Work out the finished part from the listing and answer in its coordinate system (mm). Face numbers are marked on the shaded views. A direction names the side the tool comes from. Coordinates: 2 decimals unless noted, no trailing zeros. Order: outer loops, then holes, each group sorted by start corner. A loop starts at its lowest first (then second) coordinate and runs counter-clockwise, first axis right, second up. Notation, with made-up numbers: (88.5, -32.5) -> (112.5, -32.5) arc R32 ccw to (112.5, -0.5) -> close; hole circle Ø5 at (88.5, 47.5). An arc over 180 degrees is marked (long way). Answer as CSV lines item,"result". Start each with the question number.
Item 1: Section B-B (z = 1.25) is taken. Write down the section's boundary in (x, y).
Item 2: Section C-C (x = 3.25) is taken. Write down the section's boundary in (y, z).
Item 3: Section A-A (y = 16) is taken. Write down the section's boundary in (x, z), then the cut area to 3 significant figures.
Item 4: Which of the six approach directions +Z, -Z, +X, -X, +Y, -Y give full straight-line access (tool end or side, diameter ignored) to the marked faces 4, 5, 6, 7 and 8?
Item 5: Section D-D (x = -5.25) is taken. Write down the section's boundary in (y, z), then the cut area to 3 significant figures.
Item 6: Each of these flat-tipped pins is pushed along its axis until it touches: pin 1 Ø1.5 at (y, z) = (16, 3) entering from +X; pin 2 Ø3 at (x, y) = (9, 8) entering from -Z; pin 3 Ø4 at (y, z) = (-15, -0.5) entering from -X. Where does it stop, or does it pass through?
Item 7: Straight lines are drawn through the part: L1, parallel to X at y = 13.5, z = 0.25; L2, parallel to X at y = -11.5, z = -1.75; L3, parallel to Y at x = 7.25, z = 0.5. For each, find the intervals that lie inside material, in ascending order.
Item 8: For a pull along X with two mould halves and no side action, classify the marked faces 1, 2 and 3 as pulls with the +X half, pulls with the -X half, needs draft (parallel to the pull), parting line crosses it, or undercut.
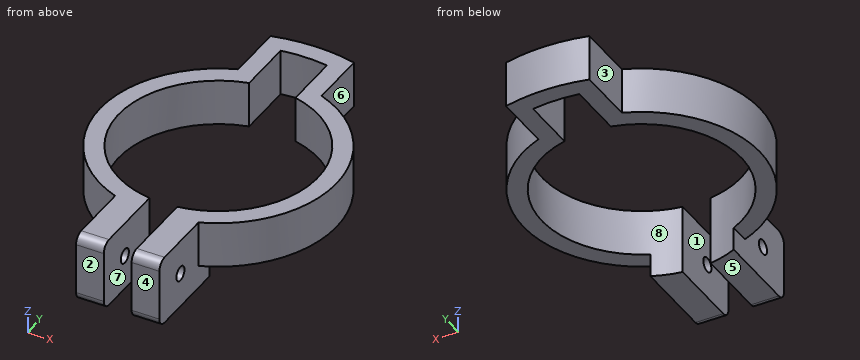
```python
from build123d import *

# Parameters (mm, degrees)
F1_DEPTH = 5
F3_DEPTH = 7.5
F5_DEPTH = 7.5
F6_R     = 1
F7_R     = 0.7847872087
F8_DEPTH = 25


with BuildPart() as f1:
    # F0 (on Top) → F1 (new body)
    with BuildSketch(Plane.XY):
        with BuildLine():
            Line((-4.5, 18.2019916493), (-4.5, 11.9294802904))
            ThreePointArc((-4.5, 11.9294802904), (0, -12.75), (4.5, 11.9294802904))
            Line((4.5, 11.9294802904), (4.5, 18.2019916493))
            ThreePointArc((4.5, 18.2019916493), (0, 18.75), (-4.5, 18.2019916493))
        make_face()
        with BuildLine():
            ThreePointArc((2.5, 10.4552618332), (0, -10.75), (-2.5, 10.4552618332))
            Line((-2.5, 10.4552618332), (-2.5, 16.5623820751))
            ThreePointArc((-2.5, 16.5623820751), (0, 16.75), (2.5, 16.5623820751))
            Line((2.5, 16.5623820751), (2.5, 10.4552618332))
        make_face(mode=Mode.SUBTRACT)
    extrude(amount=F1_DEPTH)

    # F2 (on face) → F3 (join)
    with BuildSketch(Plane.XY.offset(5)):
        with BuildLine():
            ThreePointArc((4.5, -9.7628120949), (0, -10.75), (-4.5, -9.7628120949))
            Line((-4.5, -9.7628120949), (-4.5, -11.9294802904))
            ThreePointArc((-4.5, -11.9294802904), (0, -12.75), (4.5, -11.9294802904))
            Line((4.5, -11.9294802904), (4.5, -9.7628120949))
        make_face()
        with BuildLine():
            ThreePointArc((4.5, -11.9294802904), (0, -12.75), (-4.5, -11.9294802904))
            Line((-4.5, -11.9294802904), (-4.5, -19.5))
            Line((-4.5, -19.5), (4.5, -19.5))
            Line((4.5, -19.5), (4.5, -11.9294802904))
        make_face()
    extrude(amount=-F3_DEPTH)

    # F4 (on face) → F5 (cut, through all)
    with BuildSketch(Plane.XY.offset(5)):
        with BuildLine():
            ThreePointArc((1.5, -10.644834428), (0, -10.75), (-1.5, -10.644834428))
            Line((-1.5, -10.644834428), (-1.5, -19.5))
            Line((-1.5, -19.5), (1.5, -19.5))
            Line((1.5, -19.5), (1.5, -10.644834428))
        make_face()
    extrude(amount=-F5_DEPTH, mode=Mode.SUBTRACT)

    # F6
    f6_edges = [f1.edges().sort_by_distance(p)[0] for p in [
        (-3, -19.5, 5),
        (3, -19.5, 5),
        (3, -19.5, -2.5),
        (-3, -19.5, -2.5),
    ]]
    fillet(f6_edges, radius=F6_R)

    # F7 (on face) → F8 (cut)
    with BuildSketch(Plane(origin=(-4.5, 0, 0), x_dir=(0, -1, 0), z_dir=(-1, 0, 0))):
        with Locations((15.4294802904, 1.25)):
            Circle(F7_R)
    extrude(amount=-F8_DEPTH, mode=Mode.SUBTRACT)


solid = f1.part
```
Checked values:
1,outline,"(-4.5, -19.5) -> (-1.5, -19.5) -> (-1.5, -16.21) -> (-4.5, -16.21) -> close; (-4.5, -14.64) -> (-1.5, -14.64) -> (-1.5, -10.64) arc R10.75 cw to (-2.5, 10.46) -> (-2.5, 16.56) arc R16.75 cw to (2.5, 16.56) -> (2.5, 10.46) arc R10.75 cw to (1.5, -10.64) -> (1.5, -14.64) -> (4.5, -14.64) -> (4.5, -11.93) arc R12.75 ccw to (4.5, 11.93) -> (4.5, 18.2) arc R18.75 ccw to (-4.5, 18.2) -> (-4.5, 11.93) arc R12.75 ccw to (-4.5, -11.93) -> close; (1.5, -19.5) -> (4.5, -19.5) -> (4.5, -16.21) -> (1.5, -16.21) -> close"
2,outline,"(-19.5, -1.5) arc R1 ccw to (-18.5, -2.5) -> (-10.25, -2.5) -> (-10.25, 5) -> (-18.5, 5) arc R1 ccw to (-19.5, 4) -> close; (10.25, 0) -> (18.47, 0) -> (18.47, 5) -> (10.25, 5) -> close; hole circle Ø1.57 at (-15.43, 1.25)"
3,outline,"(-4.5, 0) -> (-2.5, 0) -> (-2.5, 5) -> (-4.5, 5) -> close; (2.5, 0) -> (4.5, 0) -> (4.5, 5) -> (2.5, 5) -> close"
3,area,"20.0 mm^2"
4,face 4,"+Z, -Z, +X, -X, -Y"
4,face 5,"-Z, +X, -X, +Y, -Y"
4,face 6,"+Z, -Z, +X, +Y"
4,face 7,"+Z, -Z, -Y"
4,face 8,"+Z, -Z"
5,outline,"(-11.62, 0) -> (-9.38, 0) -> (-9.38, 5) -> (-11.62, 5) -> close; (9.38, 0) -> (11.62, 0) -> (11.62, 5) -> (9.38, 5) -> close"
5,area,"22.4 mm^2"
6,pin 1,"stops at x = 4.5"
6,pin 2,"stops at z = 0"
6,pin 3,"stops at x = -4.5"
7,L1,"x = -4.5 to -2.5, 2.5 to 4.5"
7,L2,"x = -4.5 to -1.5, 1.5 to 4.5"
7,L3,"y = -10.49 to -7.94, 7.94 to 10.49"
8,face 1,"undercut"
8,face 2,"needs draft"
8,face 3,"pulls with the -X half"
